For this review, take the finished solid that the model builds, in its own axes (mm). Face numbers are marked on the shaded views. A direction names the side the tool comes from. Coordinates: 2 decimals unless noted, no trailing zeros. Order: outer loops, then holes, each group sorted by start corner. A loop starts at its lowest first (then second) coordinate and runs counter-clockwise, first axis right, second up. Notation, with made-up numbers: M 69.25,73.25 L 80.25,73.25 A16 cw 80.25,98.25 Z; hole C -33.5,-28.5 d3. An arc over 180 degrees is marked long. Use CSV: the item, a comma, the result in double quotes.
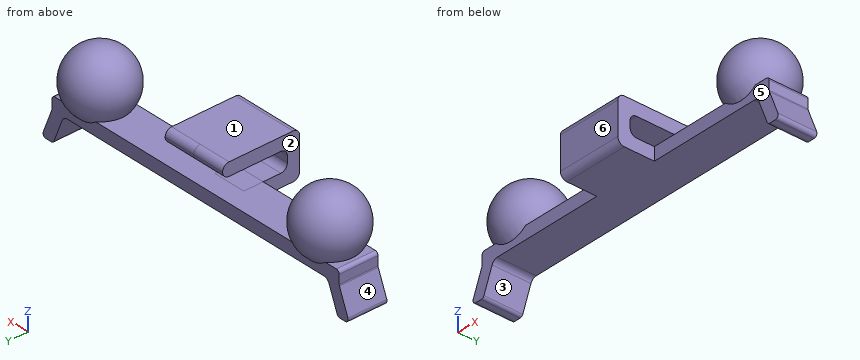
```python
from build123d import *

# Parameters (mm, degrees)
F3_DEPTH      = 3
F3_DEPTH_BACK = 3
F5_DEPTH      = 5
F5_DEPTH_BACK = 5


with BuildPart() as f2:
    # F0 (on Front) → F2 (revolve)
    with BuildSketch(Plane.XZ):
        with BuildLine():
            Line((-25, 5), (-15.0003286976, 5.0810792445))
            ThreePointArc((-15.0003286976, 5.0810792445), (-20.040703971, 10.0403752734), (-25, 5))
        make_face()
    revolve(axis=Axis((-20.0001643488, 0, 5.0405396222), (0.9999671302, 0, 0.0081079244)))

    # F0 (on Front) → F3 (join, two sides)
    with BuildSketch(Plane.XZ) as f3_sk:
        with BuildLine():
            ThreePointArc((-23.2302926299, -0.6269286958), (-22.8623688248, -0.1714255301), (-22.3024899558, 0))
            Line((-22.3024899558, 0), (0, 0))
            Line((0, 0), (0, 2))
            Line((0, 2), (-24.5, 2))
            ThreePointArc((-24.5, 2), (-24.8535533906, 1.8535533906), (-25, 1.5))
            Line((-25, 1.5), (-25, 0.0967607601))
            ThreePointArc((-25, 0.0967607601), (-25.0091076144, 0.0017625194), (-25.036098663, -0.089774892))
            Line((-25.036098663, -0.089774892), (-26.5228529957, -3.7872306599))
            ThreePointArc((-26.5228529957, -3.7872306599), (-26.4732388936, -4.2537057465), (-26.0589516587, -4.473766312))
            Line((-26.0589516587, -4.473766312), (-25.1149703996, -4.473766312))
            ThreePointArc((-25.1149703996, -4.473766312), (-24.8350309651, -4.3880535469), (-24.6510690626, -4.1603019641))
            Line((-24.6510690626, -4.1603019641), (-23.2302926299, -0.6269286958))
        make_face()
    extrude(amount=-F3_DEPTH)
    extrude(f3_sk.sketch, amount=F3_DEPTH_BACK)

    # F4: F2 across plane


with BuildPart() as f2_1:
    add(f2.part)
    add(f2.part.mirror(Plane.YZ))

    # F1 (on Right) → F5 (join, two sides)
    with BuildSketch(Plane.YZ) as f5_sk:
        with BuildLine():
            Line((-7.6333043873, 0), (0, 0))
            Line((0, 0), (0, 2))
            Line((0, 2), (-5.738430818, 2))
            ThreePointArc((-5.738430818, 2), (-6.4455375992, 2.2928932188), (-6.738430818, 3))
            Line((-6.738430818, 3), (-6.738430818, 4))
            ThreePointArc((-6.738430818, 4), (-6.4455375992, 4.7071067812), (-5.738430818, 5))
            Line((-5.738430818, 5), (2.2644215971, 5))
            ThreePointArc((2.2644215971, 5), (2.9715283783, 5.2928932188), (3.2644215971, 6))
            ThreePointArc((3.2644215971, 6), (2.9715283783, 6.7071067812), (2.2644215971, 7))
            Line((2.2644215971, 7), (-7.6333043873, 7))
            ThreePointArc((-7.6333043873, 7), (-8.3404111685, 6.7071067812), (-8.6333043873, 6))
            Line((-8.6333043873, 6), (-8.6333043873, 1))
            ThreePointArc((-8.6333043873, 1), (-8.3404111685, 0.2928932188), (-7.6333043873, 0))
        make_face()
    extrude(amount=F5_DEPTH)
    extrude(f5_sk.sketch, amount=-F5_DEPTH_BACK)


solid = f2_1.part
```
Item 1: Add section B-B on z = -1.75. State the section outline as (x, y) points.
Solutions:
outline,"M -25.7,-3 L -23.68,-3 L -23.68,3 L -25.7,3 Z; M 23.68,-3 L 25.7,-3 L 25.7,3 L 23.68,3 Z"
Item 2: Add section A-A on y = 1.5. State the section outline as (x, z) points.
Solutions:
outline,"M -26.52,-3.79 A0.5 ccw -26.06,-4.47 L -25.11,-4.47 A0.5 ccw -24.65,-4.16 L -23.23,-0.63 A1 cw -22.3,0 L 22.3,0 A1 cw 23.23,-0.63 L 24.65,-4.16 A0.5 ccw 25.11,-4.47 L 26.06,-4.47 A0.5 ccw 26.52,-3.79 L 25.04,-0.09 A0.5 cw 25,0.1 L 25,1.5 A0.5 ccw 24.5,2 L 23.68,2 A4.77 ccw long 16.33,2 L -16.33,2 A4.77 ccw long -23.68,2 L -24.5,2 A0.5 ccw -25,1.5 L -25,0.1 A0.5 cw -25.04,-0.09 Z; M -5,5 L 5,5 L 5,7 L -5,7 Z"
Item 3: For the marked faces 1, 2 and 3, list the 3-axis set-ups (+Z, -Z, +X, -X, +Y, -Y) from which the entire face can be reached by the end or side of a thin tool; tool diameter is ignored.
Solutions:
face 1,"+Z, +Y, -Y"
face 2,"+Z, -Y"
face 3,"-Z, +Y, -Y"
Item 4: Draft analysis for pull direction X (two halves, no side actions). For the marked faces 4, 5 and 6, state which applies: released by +X, released by -X, zero draft, split by the parting line, or undercut.
Solutions:
face 4,"released by -X"
face 5,"undercut"
face 6,"zero draft"
Item 5: To check wall thickness, follow line 1 along X through (y, z) = (-1, 6.25); line 2 along Y through (x, z) = (-13.5, 1); line 3 along X through (y, z) = (-7, 4.5). State the ranges of each line that lie inside material, in increasing order. Write a range as [from, to].
Solutions:
line 1,"[-24.75, -15.25], [-5, 5], [15.25, 24.75]"
line 2,"[-3, 3]"
line 3,"[-5, 5]"
Item 6: Add section C-C on x = -16. State the section outline as (y, z) points, and give its area (3 significant figures).
Solutions:
outline,"M -3,0 L 3,0 L 3,2 L -3,2 Z; C 0,5.04 d6"
area,"40.3 mm^2"
Item 7: Add section D-D on x = 3.5. State the section outline as (y, z) points, and give its area (3 significant figures).
Solutions:
outline,"M -8.63,1 A1 ccw -7.63,0 L 3,0 L 3,2 L -5.74,2 A1 cw -6.74,3 L -6.74,4 A1 cw -5.74,5 L 2.26,5 A1 ccw 2.26,7 L -7.63,7 A1 ccw -8.63,6 Z"
area,"52.3 mm^2"
Item 8: Clearance check with flat-ended pins moving along their axes: pin 1 Ø8 at (x, y) = (-2, -0.5) entering from +Z; pin 2 Ø1 at (x, y) = (-11.5, -2) entering from +Z; pin 3 Ø1.1 at (x, z) = (3.5, 3.5) entering from +Y. State where each tip first meets the part, or that it passes through.
Solutions:
pin 1,"z = 7"
pin 2,"z = 2"
pin 3,"y = -6.74"
